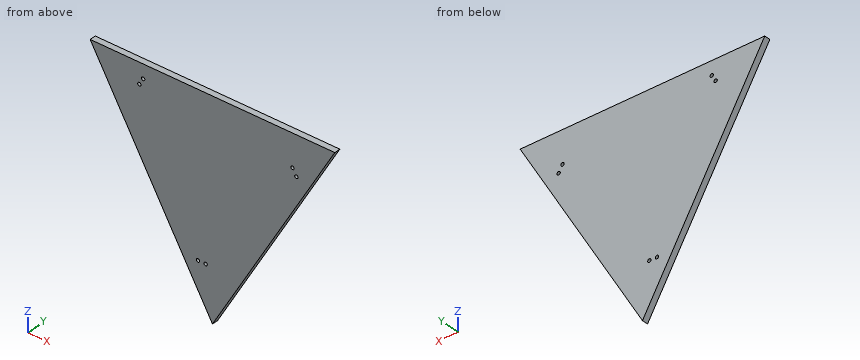
from build123d import *

# Parameters (mm, degrees)
BOSS_EXTRUDE1_DEPTH = 6.35
SKETCH2_R           = 1.7272
CUT_EXTRUDE1_DEPTH  = 195.099602868


with BuildPart() as part:
    # Sketch1 → Boss-Extrude1 (new body)
    with BuildSketch(Plane(origin=(0, 0, 0), x_dir=(1, 0, 0), z_dir=(0, 1, 0))):
        Polygon((0, 146.646968374), (-127, -73.323484187), (127, -73.323484187), align=None)
    extrude(amount=BOSS_EXTRUDE1_DEPTH)

    # Sketch2 → Cut-Extrude1 (cut, through all)
    with BuildSketch(Plane(origin=(0, 6.35, 0), x_dir=(1, 0, 0), z_dir=(0, 1, 0))):
        with Locations(Location((83.080121807, -39.724771067, 0), (0, 0, 270))):
            Circle(SKETCH2_R)
        with Locations(Location((87.042521807, -32.861692947, 0), (0, 0, 270))):
            Circle(SKETCH2_R)
        with Locations(Location((-75.942721807, -52.087110501, 0), (0, 0, 270))):
            Circle(SKETCH2_R)
        with Locations(Location((-71.980321807, -58.950188621, 0), (0, 0, 270))):
            Circle(SKETCH2_R)
        with Locations(Location((-7.1374, 91.811881567, 0), (0, 0, 270))):
            Circle(SKETCH2_R)
        with Locations(Location((-15.0622, 91.811881567, 0), (0, 0, 270))):
            Circle(SKETCH2_R)
    extrude(amount=-CUT_EXTRUDE1_DEPTH, mode=Mode.SUBTRACT)


solid = part.part
Model file for the job. Use its own axes, mm. Coordinates: 2 decimals unless noted, no trailing zeros. Order: outer loops, then holes, each group sorted by start corner. A loop starts at its lowest first (then second) coordinate and runs counter-clockwise, first axis right, second up. Notation, with made-up numbers: (-32.5, 62.25) -> (15.5, 62.25) arc R22 ccw to (15.5, 77.25) -> close; hole circle Ø5 at (-34.75, 12). An arc over 180 degrees is marked (long way). Return JSON: item names as keys, results as strings. Group by question number.
Item 1: Saw through at A-A on y = 1. Write the cut outline in (x, z).
Item 2: Saw through at C-C on z = -27. Write the cut outline in (x, y).
Item 3: Wall check: line 1 along Z through (x, y) = (98, 1.5); line 2 along Z through (x, y) = (88, 1.25); line 3 along Z through (x, y) = (-81.5, 2.5). Give the ranges that are in metal, low to high. Write a range as [from, to].
Item 4: Flat gauge pins, fed straight in: P1, Ø3, axis at x = -7.14, z = -91.81, coming from the +Y side; P2, Ø1, axis at x = -55.5, y = 3, coming from the -Z side; P3, Ø1, axis at y = 2.5, z = -59.5, coming from the -X side. Where does each tip first touch, or does it go through?
Item 5: Saw through at B-B on x = -27.5. Write the cut outline in (y, z).
Values found:
{
 "1": {"outline": "(-127, 73.32) -> (0, -146.65) -> (127, 73.32) -> close; hole circle Ø3.45 at (-75.94, 52.09); hole circle Ø3.45 at (-71.98, 58.95); hole circle Ø3.45 at (-15.06, -91.81); hole circle Ø3.45 at (-7.14, -91.81); hole circle Ø3.45 at (83.08, 39.72); hole circle Ø3.45 at (87.04, 32.86)"},
 "2": {"outline": "(-69.08, 0) -> (69.08, 0) -> (69.08, 6.35) -> (-69.08, 6.35) -> close"},
 "3": {"line 1": "z = [23.09, 73.32]", "line 2": "z = [5.77, 31.42], [34.3, 73.32]", "line 3": "z = [-5.48, 73.32]"},
 "4": {"P1": "passes through", "P2": "stops at z = -51.38", "P3": "stops at x = -50.6"},
 "5": {"outline": "(0, -99.02) -> (6.35, -99.02) -> (6.35, 73.32) -> (0, 73.32) -> close"}
}
